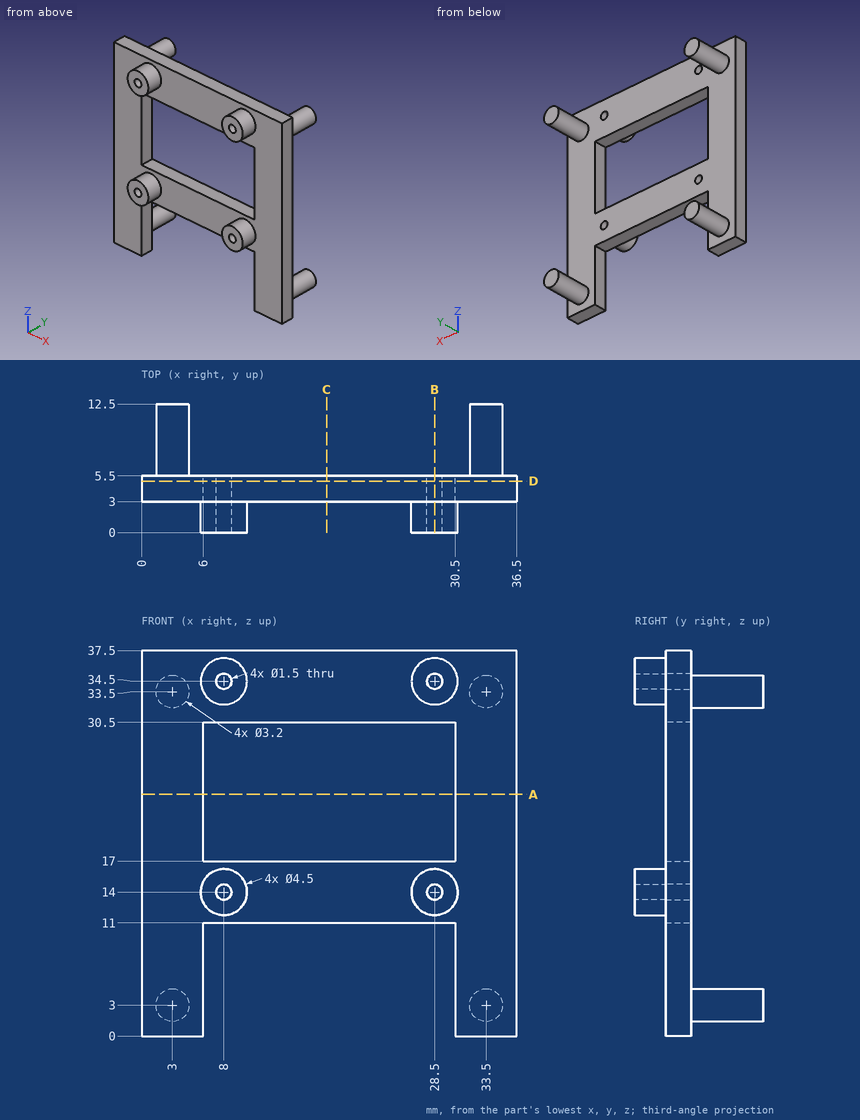
Here's the drawing with two shaded views (mm, measured from the low corner). I have some questions. Give positions to 0.01 mm unless a question says otherwise; leave off trailing zeros. Loops run counter-clockwise (first coordinate to the right, second up) from the corner with the lowest first, then second, coordinate; pieces in that order, holes last. Notation, with made-up numbers: (76, 64.25) - (95, 64.25) arc R21 ccw to (95, 70.25) - close; hole circle Ø5 at (-9.5, 40). An arc over 180 degrees is marked (long way). Return JSON: item names as keys, results as strings.
1. I want a section at D-D on y = 5. Please give me the cut outline in (x, z).
Output values:
{"outline": "(0, 0) - (6, 0) - (6, 11) - (30.5, 11) - (30.5, 0) - (36.5, 0) - (36.5, 37.5) - (0, 37.5) - close; hole (6, 17) - (30.5, 17) - (30.5, 30.5) - (6, 30.5) - close; hole circle Ø1.5 at (8, 14); hole circle Ø1.5 at (8, 34.5); hole circle Ø1.5 at (28.5, 14); hole circle Ø1.5 at (28.5, 34.5)"}
2. I want a section at A-A on z = 23.5. Please give me the cut outline in (x, y).
Output values:
{"outline": "(0, 3) - (6, 3) - (6, 5.5) - (0, 5.5) - close; (30.5, 3) - (36.5, 3) - (36.5, 5.5) - (30.5, 5.5) - close"}
3. I want a section at B-B on x = 28.5. Please give me the cut outline in (y, z), and give its area (3 significant figures).
Output values:
{"outline": "(0, 11.75) - (3, 11.75) - (3, 11) - (5.5, 11) - (5.5, 13.25) - (0, 13.25) - close; (0, 14.75) - (5.5, 14.75) - (5.5, 17) - (3, 17) - (3, 16.25) - (0, 16.25) - close; (0, 32.25) - (3, 32.25) - (3, 30.5) - (5.5, 30.5) - (5.5, 33.75) - (0, 33.75) - close; (0, 35.25) - (5.5, 35.25) - (5.5, 37.5) - (3, 37.5) - (3, 36.75) - (0, 36.75) - close", "area": "43.0 mm²"}
4. If I drill on line 1 (Z direction, x = 8, y = 3.9); line 2 (X direction, y = 1.3, z = 34.5); line 3 (Z direction, x = 8, y = 2.3), over which ranges is the centre line in solid material (lowest first)?
Output values:
{"line 1": "z = 11 to 13.25, 14.75 to 17, 30.5 to 33.75, 35.25 to 37.5", "line 2": "x = 5.75 to 7.25, 8.75 to 10.25, 26.25 to 27.75, 29.25 to 30.75", "line 3": "z = 11.75 to 13.25, 14.75 to 16.25, 32.25 to 33.75, 35.25 to 36.75"}
5. I want a section at C-C on x = 18. Please give me the cut outline in (y, z), and give its area (3 significant figures).
Output values:
{"outline": "(3, 11) - (5.5, 11) - (5.5, 17) - (3, 17) - close; (3, 30.5) - (5.5, 30.5) - (5.5, 37.5) - (3, 37.5) - close", "area": "32.5 mm²"}
6. I'm going to push flat-ended pins straight in: pin 1 Ø1.2 at (x, y) = (13.5, 4) entering from -Z; pin 2 Ø8 at (x, z) = (19.5, 8.5) entering from +Y; pin 3 Ø3 at (x, z) = (30.5, 22) entering from -Y. Where does each tip first touch, or does it pass through?
Output values:
{"pin 1": "stops at z = 11", "pin 2": "stops at y = 5.5", "pin 3": "stops at y = 3"}
